Study the drawing (mm; zero at the part's minimum x, y, z) and answer. A direction names the side the tool comes from. Give positions to 0.01 mm unless a question says otherwise; leave off trailing zeros. Order: outer loops, then holes, each group sorted by start corner. A loop starts at its lowest first (then second) coordinate and runs counter-clockwise, first axis right, second up.
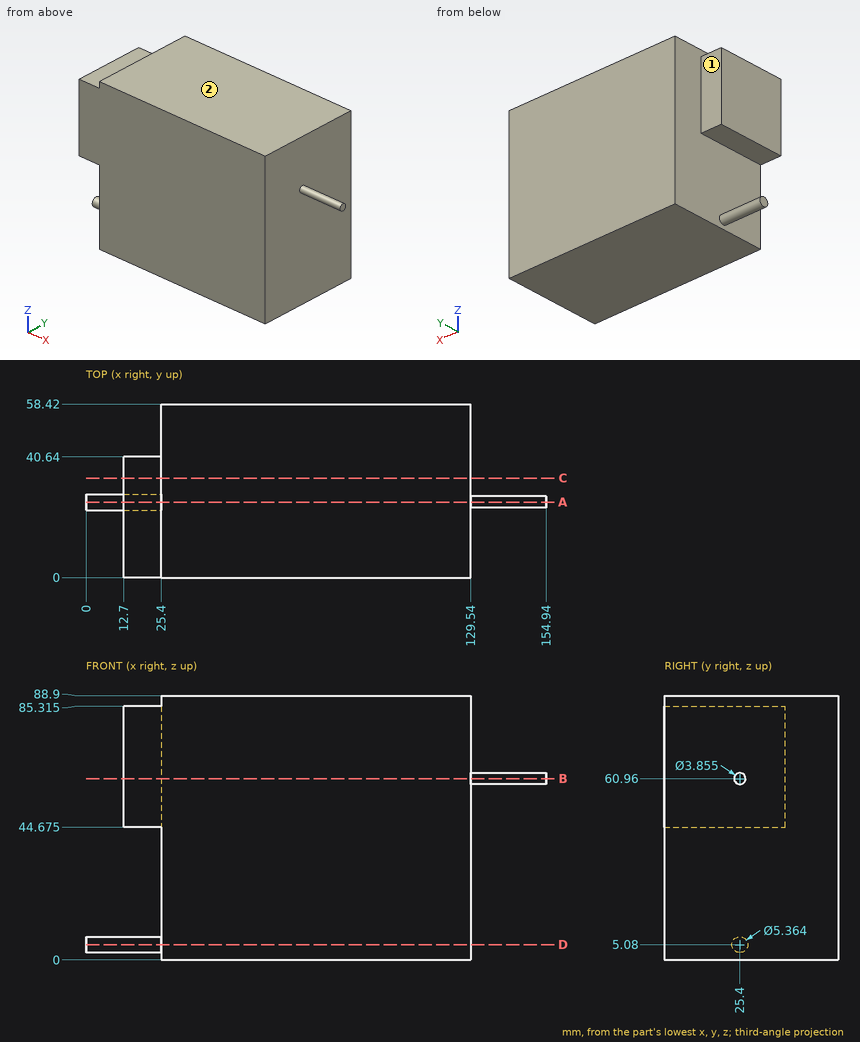
1) Find section B-B (z = 60.96). Write down the section's boundary in (x, y), then the cut area to 3 significant figures.
Geometry says:
outline: (12.7, 0) - (129.54, 0) - (129.54, 23.47) - (154.94, 23.47) - (154.94, 27.33) - (129.54, 27.33) - (129.54, 58.42) - (25.4, 58.42) - (25.4, 40.64) - (12.7, 40.64) - close
area: 6,700 mm2
2) Find section A-A (y = 25.4). Write down the section's boundary in (x, z) (1 decimal), then the cut area to 3 significant figures.
Geometry says:
outline: (0, 2.4) - (25.4, 2.4) - (25.4, 0) - (129.5, 0) - (129.5, 59) - (154.9, 59) - (154.9, 62.9) - (129.5, 62.9) - (129.5, 88.9) - (25.4, 88.9) - (25.4, 85.3) - (12.7, 85.3) - (12.7, 44.7) - (25.4, 44.7) - (25.4, 7.8) - (0, 7.8) - close
area: 10,000 mm2
3) Find section D-D (z = 5.08). Write down the section's boundary in (x, y), then the cut area to 3 significant figures.
Geometry says:
outline: (0, 22.72) - (25.4, 22.72) - (25.4, 0) - (129.54, 0) - (129.54, 58.42) - (25.4, 58.42) - (25.4, 28.08) - (0, 28.08) - close
area: 6,220 mm2
4) Straight lines are drawn through the part: probe 1 along X at (y, z) = (50, 40); probe 2 along X at (y, z) = (6.5, 47.5); probe 3 along Z at (x, y) = (20, 32) (1 decimal). For each, find the intervals that lie inside material, in ascending order.
Geometry says:
probe 1: x = 25.4 to 129.54
probe 2: x = 12.7 to 129.54
probe 3: z = 44.7 to 85.3
5) A tool of negligible diameter and unlimited length cuts with its end or side. For the marked faces 1 and 2, from which of +Z, -Z, +X, -X, +Y, -Y can it reach the whole face along a straight path? Write none if from no direction.
Geometry says:
face 1: +Z, -Z, -X, +Y
face 2: +Z, +X, -X, +Y, -Y
6) Given P1, Ø6.5, axis at x = 18.5, z = 59, coming from the +Y side; P2, Ø5, axis at y = 32.5, z = 35.5, coming from the -X side; P3, Ø4, axis at x = 17.5, y = 22, coming from the -Z side, each flat-ended and moving along its own axis, determine where each tip first touches the part or whether it passes through.
Geometry says:
P1: stops at y = 40.64
P2: stops at x = 25.4
P3: stops at z = 2.79
7) Find section C-C (y = 33.5). Write down the section's boundary in (x, z) (1 decimal).
Geometry says:
outline: (12.7, 44.7) - (25.4, 44.7) - (25.4, 0) - (129.5, 0) - (129.5, 88.9) - (25.4, 88.9) - (25.4, 85.3) - (12.7, 85.3) - close
